Here's how the part is built. I have some questions about the finished solid (model axes, mm). Coordinates: 2 decimals unless noted, no trailing zeros. Order: outer loops, then holes, each group sorted by start corner. A loop starts at its lowest first (then second) coordinate and runs counter-clockwise, first axis right, second up. Notation, with made-up numbers: (3, -6) - (61, -6) arc R23 ccw to (61, 15) - close; hole circle Ø8 at (81, -29.75). An arc over 180 degrees is marked (long way). Answer in a Markdown table with one row per item. Add a question column.
Item 1: Thinking about a two-plate mould opening in X: for faces 1 (the flat face through (3, 3, 3.5)), 2 (the conical face through (-1.329, 5.984, 2.892)), 3 (the cylindrical face through (-3.746, -0.165, 1.726)), which applies, +X half, -X half, draft (parallel to the pull), parting line (faces both ways), or undercut?
Item 2: I want a section at B-B (z = 2.7). Please give me the cut outline in (x, y).
Item 3: If I drill on line 1 along X through (y, z) = (0, 2.55); line 2 along X through (y, z) = (0, 0.6), over which ranges is the centre line in solid material (lowest first)? Write a range as from..to.
Item 4: I want a section at A-A (x = 0). Please give me the cut outline in (y, z).
Item 5: I want a section at C-C (z = 1.15). Please give me the cut outline in (x, y), plus the area to 3 significant figures.
Item 6: Will these pins go through, and if not, where does the flat tip stop? pin 1 Ø1 at (y, z) = (-2.5, 0.5) entering from -X; pin 2 Ø2 at (x, z) = (-1, 1) entering from -Y.
Autodesk Fusion 360 part; units mm, degrees
sketch "Esquisse1" plane through (0, 0, 0) normal (0, 0, 1) x (1, 0, 0)
  circle A0 centre (0, 0) radius 6.75
  dimension "d1" = 13.5
extrude "Extrusion1" add sketch "Esquisse1" along normal blind 3.5 makes body 1
sketch "Esquisse2" plane through (0, 0, 3.5) normal (0, 0, 1) x (-1, 0, 0)
  circle A0 centre (0, 0) radius 6.75
  circle A1 centre (0, 0) radius 6
  dimension "d4" = 12
loft "Lissage1" add profiles "Esquisse1", "Esquisse2" section 1 section 2 contours A1 separate body makes body 2
sketch "Esquisse3" plane through (0, 0, 0) normal (0, 0, 1) x (1, 0, 0)
  circle A0 centre (0, 0) radius 3.375
  dimension "d5" = 6.75
extrude "Extrusion2" cut sketch "Esquisse3" along normal blind 33 bodies 2
sketch "Esquisse4" plane through (0, 0, 0) normal (0, 0, 1) x (1, 0, 0)
  circle A0 centre (0, 0) radius 3.75
  dimension "d8" = 7.5
extrude "Extrusion3" cut sketch "Esquisse4" along normal blind 23 bodies 2
hidden bodies 1
Values follow:
| question | item | result |
|---|---|---|
| 1 | face 1 | draft |
| 1 | face 2 | parting line |
| 1 | face 3 | undercut |
| 2 | outline | circle Ø12.34 at (0, 0); hole circle Ø7.5 at (0, 0) |
| 3 | line 1 | x = -6.2..-3.75, 3.75..6.2 |
| 3 | line 2 | x = -6.62..-3.75, 3.75..6.62 |
| 4 | outline | (-6.75, 0) - (-3.75, 0) - (-3.75, 3.5) - (-6, 3.5) - close; (3.75, 0) - (6.75, 0) - (6, 3.5) - (3.75, 3.5) - close |
| 5 | outline | circle Ø13.01 at (0, 0); hole circle Ø7.5 at (0, 0) |
| 5 | area | 88.7 mm^2 |
| 6 | pin 1 | stops at x = -6.37 |
| 6 | pin 2 | stops at y = -6.71 |
